For this review, take the finished solid that the model builds, in its own axes (mm). Face numbers are marked on the shaded views. A direction names the side the tool comes from. Give positions to 0.01 mm unless a question says otherwise; leave off trailing zeros. Order: outer loops, then holes, each group sorted by start corner. A loop starts at its lowest first (then second) coordinate and runs counter-clockwise, first axis right, second up.
from build123d import *

# Parameters (mm, degrees)
BOSS_EXTRU_1_DEPTH      = 36
ENL_V_MAT_EXTRU_1_DEPTH = 36
ENL_V_MAT_EXTRU_2_DEPTH = 36
CHANFREIN1_SIZE         = 1


with BuildPart() as part:
    # Esquisse1 → Boss.-Extru.1 (new body)
    with BuildSketch(Plane.XY):
        Polygon((0, 0), (0, 150), (110, 150), (110, 141), (9, 141), (9, 0), align=None)
    extrude(amount=BOSS_EXTRU_1_DEPTH)

    # Esquisse2 → Enlèv. mat.-Extru.1 (cut)
    with BuildSketch(Plane.ZY):
        with BuildLine():
            Line((23, 125), (23, 35))
            ThreePointArc((23, 35), (18, 30), (13, 35))
            Line((13, 35), (13, 125))
            ThreePointArc((13, 125), (18, 130), (23, 125))
        make_face()
    extrude(amount=-ENL_V_MAT_EXTRU_1_DEPTH, mode=Mode.SUBTRACT)

    # Esquisse3 → Enlèv. mat.-Extru.2 (cut)
    with BuildSketch(Plane(origin=(0, 150, 0), x_dir=(1, 0, 0), z_dir=(0, 1, 0))):
        with BuildLine():
            Line((36, -12), (84, -12))
            ThreePointArc((84, -12), (90, -18), (84, -24))
            Line((84, -24), (36, -24))
            ThreePointArc((36, -24), (30, -18), (36, -12))
        make_face()
    extrude(amount=-ENL_V_MAT_EXTRU_2_DEPTH, mode=Mode.SUBTRACT)

    # Chanfrein1
    chanfrein1_edges = [part.edges().sort_by_distance(p)[0] for p in [
        (59.5, 141, 36),
        (0, 0, 18),
        (0, 150, 18),
        (110, 150, 18),
        (110, 141, 18),
        (9, 0, 18),
        (110, 145.5, 36),
        (55, 150, 36),
        (0, 75, 36),
        (9, 130, 18),
        (9, 80, 23),
        (9, 30, 18),
        (9, 80, 13),
        (0, 130, 18),
        (0, 80, 13),
        (0, 30, 18),
        (0, 80, 23),
        (4.5, 0, 36),
        (30, 141, 18),
        (60, 141, 12),
        (90, 141, 18),
        (60, 141, 24),
        (30, 150, 18),
        (60, 150, 24),
        (90, 150, 18),
        (60, 150, 12),
        (0, 75, 0),
        (55, 150, 0),
        (110, 145.5, 0),
        (9, 70.5, 36),
        (59.5, 141, 0),
        (9, 70.5, 0),
        (4.5, 0, 0),
    ]]
    chamfer(chanfrein1_edges, length=CHANFREIN1_SIZE)


solid = part.part
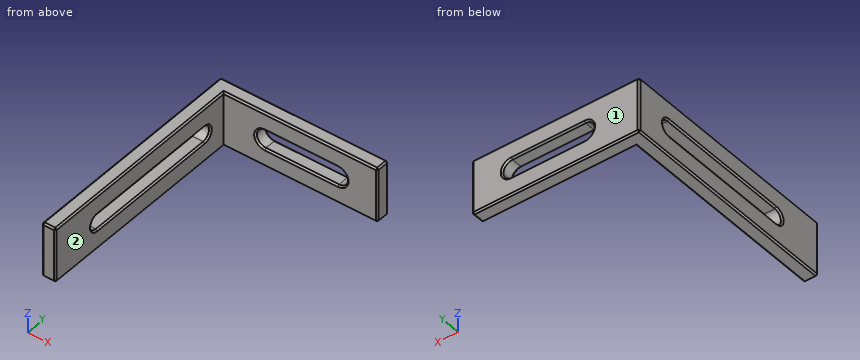
1) To check wall thickness, follow line 1 (Z direction, x = 6, y = 124); line 2 (X direction, y = 123.5, z = 34); line 3 (Y direction, x = 99.5, z = 14.5). State the ranges of each line that lie inside material, in increasing order.
Answer sheet:
line 1: z = 0 to 13, 23 to 36
line 2: x = 0 to 9
line 3: y = 141 to 150
2) Clearance check with flat-ended pins moving along their axes: pin 1 (3 mm diameter, centred on y = 52, z = 22, fed in from +X); pin 2 (10 mm diameter, centred on y = 24.5, z = 21, fed in from +X); pin 3 (10 mm diameter, centred on x = 45.5, z = 23.5, fed in from +Y). State where each tip first meets the part, or that it passes through.
Answer sheet:
pin 1: stops at x = 8.5
pin 2: stops at x = 9
pin 3: stops at y = 150
3) We need section B-B on y = 104.5. Give the boundary of the cut face in (x, z).
Answer sheet:
outline: (0, 1) - (1, 0) - (8, 0) - (9, 1) - (9, 12) - (8, 13) - (1, 13) - (0, 12) - close; (0, 24) - (1, 23) - (8, 23) - (9, 24) - (9, 35) - (8, 36) - (1, 36) - (0, 35) - close
4) We need section C-C on z = 31.5. Give the boundary of the cut face in (x, y).
Answer sheet:
outline: (0, 1) - (1, 0) - (8, 0) - (9, 1) - (9, 141) - (109, 141) - (110, 142) - (110, 149) - (109, 150) - (1, 150) - (0, 149) - close
5) We need section A-A on x = 70.5. Give the boundary of the cut face in (y, z), then the cut area to 3 significant figures.
Answer sheet:
outline: (141, 1) - (142, 0) - (149, 0) - (150, 1) - (150, 11) - (149, 12) - (142, 12) - (141, 11) - close; (141, 25) - (142, 24) - (149, 24) - (150, 25) - (150, 35) - (149, 36) - (142, 36) - (141, 35) - close
area: 212 mm2
6) Tool access review of the marked faces 1 and 2: name each direction out of +Z, -Z, +X, -X, +Y, -Y from which nothing blocks a thin tool from reaching the whole face with its end or side.
Answer sheet:
face 1: +Z, -Z, +X, -X, +Y
face 2: +Z, -Z, +X, -Y
7) We need section D-D on x = 13.5. Give the boundary of the cut face in (y, z), then the cut area to 3 significant figures.
Answer sheet:
outline: (141, 1) - (142, 0) - (149, 0) - (150, 1) - (150, 35) - (149, 36) - (142, 36) - (141, 35) - close
area: 322 mm2
